```python
from build123d import *

# Parameters (mm, degrees)
BOSS_EXTRUDE1_DEPTH             = 2
F_4_40_TAPPED_HOLE1_D           = 2.2606
F_4_40_TAPPED_HOLE1_DEPTH       = 30
F_4_40_TAPPED_HOLE1_CSINK_D     = 4.1148
F_4_40_TAPPED_HOLE1_CSINK_ANGLE = 100
F_4_40_TAPPED_HOLE1_TIP         = 0.679152758


with BuildPart() as part:
    # Sketch1 → Boss-Extrude1 (new body)
    with BuildSketch(Plane(origin=(0, 0, 0), x_dir=(1, 0, 0), z_dir=(0, 1, 0))):
        with BuildLine():
            Line((-6.920754264, 5), (3.079245736, 5))
            ThreePointArc((3.079245736, 5), (8.079245736, 0), (3.079245736, -5))
            Line((3.079245736, -5), (-6.920754264, -5))
            ThreePointArc((-6.920754264, -5), (-11.920754264, 0), (-6.920754264, 5))
        make_face()
    extrude(amount=BOSS_EXTRUDE1_DEPTH)

    # #4-40 Tapped Hole1
    with Locations(Plane(origin=(28.793519494, 0, 54.352929604), x_dir=(-0.6824480483722141, 0, -0.7309341018675735), z_dir=(0, -1, 0))):
        with Locations((57.277065725, 18.297611137)):
            CounterSinkHole(F_4_40_TAPPED_HOLE1_D / 2, F_4_40_TAPPED_HOLE1_CSINK_D / 2, depth=F_4_40_TAPPED_HOLE1_DEPTH, counter_sink_angle=F_4_40_TAPPED_HOLE1_CSINK_ANGLE)
            with Locations((0, 0, -(F_4_40_TAPPED_HOLE1_DEPTH + F_4_40_TAPPED_HOLE1_TIP / 2))):  # 118° drill point
                Cone(0, F_4_40_TAPPED_HOLE1_D / 2, F_4_40_TAPPED_HOLE1_TIP, mode=Mode.SUBTRACT)


solid = part.part
```
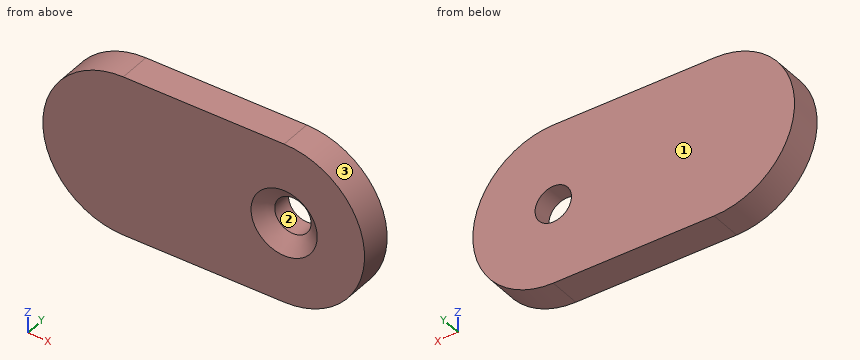
Design review of the part built by this model. Coordinates are the model's own, in mm. Face numbers are marked on the shaded views. Give positions to 0.01 mm unless a question says otherwise; leave off trailing zeros. Write each loop counter-clockwise with the first axis right and the second up, starting at its lowest first coordinate (ties: lowest second). Pieces come first, ordered by that corner, then holes. Notation, with made-up numbers: (78.25, 40) -> (124.25, 40) arc R23 ccw to (124.25, 74) -> close; hole circle Ø11 at (-5.75, -34.5). An arc over 180 degrees is marked (long way). Answer in a Markdown table with one row per item.
(1) Consider section D-D (y = 0.45). State the section outline as (x, z) points, then the cut area to 3 significant figures.
Results:
| item | result |
|---|---|
| outline | (-6.92, -5) -> (3.08, -5) arc R5 ccw to (3.08, 5) -> (-6.92, 5) arc R5 ccw to start; hole circle Ø3.04 at (3.08, 0) |
| area | 171 mm2 |
(2) Consider section C-C (x = 6). State the section outline as (y, z) points, then the cut area to 3 significant figures.
Results:
| item | result |
|---|---|
| outline | (0, -4.06) -> (2, -4.06) -> (2, 4.06) -> (0, 4.06) -> close |
| area | 16.2 mm2 |
(3) To check wall thickness, follow probe 1 along X at (y, z) = (1.45, 0); probe 2 along X at (y, z) = (1.6, 1); probe 3 along Z at (x, y) = (-10, 1.1). State the ranges of each line that lie inside material, in increasing order.
Results:
| item | result |
|---|---|
| probe 1 | -11.92 to 1.95, 4.21 to 8.08 |
| probe 2 | -11.82 to 2.55, 3.61 to 7.98 |
| probe 3 | -3.94 to 3.94 |
(4) Mouldability with a two-part tool opening along Z and no side actions: class the marked faces 1, 2 and 3 as +Z half, -Z half, draft (parallel to the pull), parting line (faces both ways), or undercut.
Results:
| item | result |
|---|---|
| face 1 | draft |
| face 2 | undercut |
| face 3 | parting line |
(5) Consider section B-B (y = 1.75). State the section outline as (x, z) points.
Results:
| item | result |
|---|---|
| outline | (-6.92, -5) -> (3.08, -5) arc R5 ccw to (3.08, 5) -> (-6.92, 5) arc R5 ccw to start; hole circle Ø2.26 at (3.08, 0) |
(6) Clearance check with a flat-ended pin moving along its axis: pin 1 (3 mm diameter, centred on x = 3.08, z = 0, fed in from -Y). State where the tip first meets the part, or that it passes through.
Results:
| item | result |
|---|---|
| pin 1 | y = 0.47 |
(7) Consider section A-A (z = 0). State the section outline as (x, y) points, then the cut area to 3 significant figures.
Results:
| item | result |
|---|---|
| outline | (-11.92, 0) -> (1.02, 0) -> (1.95, 0.78) -> (1.95, 2) -> (-11.92, 2) -> close; (4.21, 0.78) -> (5.14, 0) -> (8.08, 0) -> (8.08, 2) -> (4.21, 2) -> close |
| area | 34.8 mm2 |
